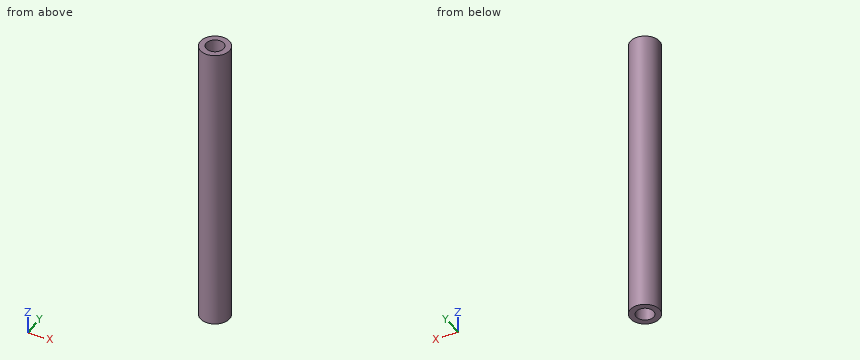
from build123d import *

# Parameters (mm, degrees)
SKETCH1_R           = 2.5
BOSS_EXTRUDE2_DEPTH = 50
SKETCH2_R           = 1.5
CUT_EXTRUDE1_DEPTH  = 6
CUT_EXTRUDE2_START  = -6
SKETCH3_R           = 1.5
CUT_EXTRUDE2_DEPTH  = 6


with BuildPart() as part:
    # Sketch1 → Boss-Extrude2 (new body)
    with BuildSketch(Plane.XY):
        Circle(SKETCH1_R)
    extrude(amount=BOSS_EXTRUDE2_DEPTH)

    # Sketch2 → Cut-Extrude1 (cut)
    with BuildSketch(Plane.XY.offset(50)):
        Circle(SKETCH2_R)
    extrude(amount=-CUT_EXTRUDE1_DEPTH, mode=Mode.SUBTRACT)

    # Sketch3 → Cut-Extrude2 (cut)
    with BuildSketch(Plane(origin=(0, 0, 0), x_dir=(-1, 0, 0), z_dir=(0, 0, -1)).offset(CUT_EXTRUDE2_START)):
        with Locations(Location((0, 0, 0), (0, 0, 180))):
            Circle(SKETCH3_R)
    extrude(amount=CUT_EXTRUDE2_DEPTH, mode=Mode.SUBTRACT)


solid = part.part
Build history of the part. All positions in model axes, mm. Give positions to 0.01 mm unless a question says otherwise; leave off trailing zeros. Order: outer loops, then holes, each group sorted by start corner. A loop starts at its lowest first (then second) coordinate and runs counter-clockwise, first axis right, second up. Notation, with made-up numbers: M 19,-3 L 52,-3 A22 cw 52,34 Z; hole C 52,1.5 d3. An arc over 180 degrees is marked long. Use one line per item in the form item = value.
1) Drop flat-ended pins along their axis: pin 1 (1.5 mm diameter, centred on x = 0, y = 0.5, fed in from -Z); pin 2 (1 mm diameter, centred on y = -2, z = 12, fed in from +X); pin 3 (1.5 mm diameter, centred on y = -1.5, z = 36.5, fed in from -X); pin 4 (1.5 mm diameter, centred on x = -0.5, z = 13, fed in from +Y). Give the stop position or say it passes through.
Calculated:
pin_1 = 6
pin_2 = 2
pin_3 = -2.38
pin_4 = 2.5
2) Saw through at C-C (z = 41.5). Give the cut face in (x, y).
Calculated:
outline = C 0,0 d5
3) Probe probe 1 along Y at (x, z) = (0, 48.3); probe 2 along Z at (x, y) = (-0.65, -0.8); probe 3 along X at (y, z) = (0.1, 13.5). List the from-to ranges inside material, lowest first.
Calculated:
probe_1 = -2.5 to -1.5, 1.5 to 2.5
probe_2 = 6 to 44
probe_3 = -2.5 to 2.5
4) Saw through at A-A (y = 0). Give the cut face in (x, z).
Calculated:
outline = M -2.5,0 L -1.5,0 L -1.5,6 L 1.5,6 L 1.5,0 L 2.5,0 L 2.5,50 L 1.5,50 L 1.5,44 L -1.5,44 L -1.5,50 L -2.5,50 Z
